```python
from build123d import *

# Parameters (mm, degrees)
SKETCH3_W           = 100
SKETCH3_H           = 63
BOSS_EXTRUDE1_DEPTH = 3
BOSS_EXTRUDE2_START = -3
SKETCH5_W           = 8
SKETCH5_H           = 6
BOSS_EXTRUDE2_DEPTH = 3
FILLET2_R           = 2
CUT_EXTRUDE1_DEPTH  = 3
CUT_EXTRUDE2_START  = -3
CUT_EXTRUDE2_DEPTH  = 3
CUT_EXTRUDE3_START  = -3
SKETCH8_W           = 39.05
SKETCH8_H           = 6
CUT_EXTRUDE3_DEPTH  = 3
SKETCH9_R           = 1.5
CUT_EXTRUDE4_DEPTH  = 10
FILL_PATTERN1_DEPTH = 3


# Read off the part's stored shape, not the designer's step: Cut-Extrude2, Fill Pattern1
with BuildPart() as part:
    # Sketch3 → Boss-Extrude1 (new body)
    with BuildSketch(Plane.XY):
        Rectangle(SKETCH3_W, SKETCH3_H)
    extrude(amount=BOSS_EXTRUDE1_DEPTH)

    # Sketch5 → Boss-Extrude2 (add)
    with BuildSketch(Plane(origin=(0, 0, 0), x_dir=(-1, 0, 0), z_dir=(0, 0, -1)).offset(BOSS_EXTRUDE2_START)):
        with Locations((-54, -28.5)):
            Rectangle(SKETCH5_W, SKETCH5_H)
        Polygon((-58, 29.5), (-50, 29.5), (-50, 31.5), (-48, 31.5), (-48, 35.5), (-58, 35.5), align=None)
        with Locations((54, -28.5)):
            Rectangle(SKETCH5_W, SKETCH5_H)
        Polygon((48, 35.5), (48, 31.5), (50, 31.5), (50, 29.5), (58, 29.5), (58, 35.5), align=None)
    extrude(amount=BOSS_EXTRUDE2_DEPTH)

    # Fillet2
    fillet2_edges = [part.edges().sort_by_distance(p)[0] for p in [
        (48, 35.5, 1.5),
        (58, 35.5, 1.5),
        (58, 29.5, 1.5),
        (50, 29.5, 1.5),
        (58, -31.5, 1.5),
        (58, -25.5, 1.5),
        (50, -25.5, 1.5),
        (-58, -31.5, 1.5),
        (-58, -25.5, 1.5),
        (-50, -25.5, 1.5),
        (-50, 29.5, 1.5),
        (-58, 29.5, 1.5),
        (-58, 35.5, 1.5),
        (-48, 35.5, 1.5),
        (-48, 31.5, 1.5),
        (48, 31.5, 1.5),
    ]]
    fillet(fillet2_edges, radius=FILLET2_R - 0.0001)  # a hair under: the kernel refuses the full size

    # Sketch6 → Cut-Extrude1 (cut)
    with BuildSketch(Plane.XY.offset(3)):
        with BuildLine():
            ThreePointArc((6.45, -3.15), (4.682233047, -3.882233047), (3.95, -5.65))
            Line((3.95, -5.65), (11.45, -5.65))
            Line((11.45, -5.65), (11.45, -3.15))
            Line((11.45, -3.15), (6.45, -3.15))
        make_face()
        with BuildLine():
            Line((11.45, -3.15), (11.45, -5.65))
            Line((11.45, -5.65), (18.95, -5.65))
            ThreePointArc((18.95, -5.65), (18.217766953, -3.882233047), (16.45, -3.15))
            Line((16.45, -3.15), (11.45, -3.15))
        make_face()
        with BuildLine():
            Line((18.95, -5.65), (11.45, -5.65))
            Line((11.45, -5.65), (11.45, -8.15))
            Line((11.45, -8.15), (16.45, -8.15))
            ThreePointArc((16.45, -8.15), (18.217766953, -7.417766953), (18.95, -5.65))
        make_face()
        with BuildLine():
            Line((11.45, -5.65), (3.95, -5.65))
            ThreePointArc((3.95, -5.65), (4.682233047, -7.417766953), (6.45, -8.15))
            Line((6.45, -8.15), (11.45, -8.15))
            Line((11.45, -8.15), (11.45, -5.65))
        make_face()
    extrude(amount=-CUT_EXTRUDE1_DEPTH, mode=Mode.SUBTRACT)

    # Cut-Extrude2 outline → Cut-Extrude2 (cut)
    with BuildSketch(Plane.XY.offset(3).offset(CUT_EXTRUDE2_START)):
        with BuildLine():
            Line((-11.2, 8.796347875), (-20.2, 8.796347875))
            ThreePointArc((-20.2, 8.796347875), (-22.2, 6.796347875), (-20.2, 4.796347875))
            Line((-20.2, 4.796347875), (1.9, 4.796347875))
            ThreePointArc((1.9, 4.796347875), (3.9, 6.796347875), (1.9, 8.796347875))
            Line((1.9, 8.796347875), (-11.19861108, 8.796347875))
            Line((-11.19861108, 8.796347875), (-11.2, 8.796347875))
        make_face()
    extrude(amount=CUT_EXTRUDE2_DEPTH, mode=Mode.SUBTRACT)

    # Sketch8 → Cut-Extrude3 (cut)
    with BuildSketch(Plane.XY.offset(3).offset(CUT_EXTRUDE3_START)):
        with BuildLine():
            Line((4.05, 14.6), (-35, 14.6))
            Line((-35, 14.6), (-35, 8.6))
            Line((-35, 8.6), (-21.064198479, 8.6))
            ThreePointArc((-21.064198479, 8.6), (-20.643111582, 8.746643269), (-20.2, 8.796347875))
            Line((-20.2, 8.796347875), (-11.2, 8.796347875))
            Line((-11.2, 8.796347875), (-11.19861108, 8.796347392))
            Line((-11.19861108, 8.796347392), (1.9, 8.796347875))
            ThreePointArc((1.9, 8.796347875), (2.343111582, 8.746643269), (2.764198479, 8.6))
            Line((2.764198479, 8.6), (4.05, 8.6))
            Line((4.05, 8.6), (4.05, 14.6))
        make_face()
        with BuildLine():
            ThreePointArc((-35, 20.6), (-39.242640687, 18.842640687), (-41, 14.6))
            Line((-41, 14.6), (-35, 14.6))
            Line((-35, 14.6), (-35, 20.6))
        make_face()
        with BuildLine():
            Line((-35, 14.6), (-41, 14.6))
            ThreePointArc((-41, 14.6), (-39.242640687, 10.357359313), (-35, 8.6))
            Line((-35, 8.6), (-35, 14.6))
        make_face()
        with Locations((-15.475, 17.6)):
            Rectangle(SKETCH8_W, SKETCH8_H)
        with BuildLine():
            Line((4.05, 20.6), (4.05, 14.6))
            Line((4.05, 14.6), (10.05, 14.6))
            ThreePointArc((10.05, 14.6), (8.292640687, 18.842640687), (4.05, 20.6))
        make_face()
        with BuildLine():
            Line((10.05, 14.6), (4.05, 14.6))
            Line((4.05, 14.6), (4.05, 8.6))
            ThreePointArc((4.05, 8.6), (8.292640687, 10.357359313), (10.05, 14.6))
        make_face()
    extrude(amount=CUT_EXTRUDE3_DEPTH, mode=Mode.SUBTRACT)

    # Sketch9 → Cut-Extrude4 (cut)
    with BuildSketch(Plane(origin=(0, 0, 0), x_dir=(-1, 0, 0), z_dir=(0, 0, -1))):
        with Locations((-54, 32.520438715)):
            Circle(SKETCH9_R)
        with Locations((54, 32.520438715)):
            Circle(SKETCH9_R)
        with Locations((-54, -28.5)):
            Circle(SKETCH9_R)
        with Locations((54, -28.5)):
            Circle(SKETCH9_R)
    extrude(amount=-CUT_EXTRUDE4_DEPTH, mode=Mode.SUBTRACT)

    # Fill Pattern1 outline → Fill Pattern1 (cut)
    with BuildSketch(Plane.XY):
        Polygon((34.648052979, 5.68067969), (32.648052979, 9.144781305), (28.648052979, 9.144781305), (26.648052979, 5.68067969), (28.648052979, 2.216578074), (32.648052979, 2.216578074), align=None)
        Polygon((27.719849748, 17.68067969), (25.719849748, 21.144781305), (21.719849748, 21.144781305), (19.719849748, 17.68067969), (21.719849748, 14.216578074), (25.719849748, 14.216578074), align=None)
        Polygon((35.576256209, 21.144781305), (33.576256209, 17.68067969), (35.576256209, 14.216578074), (39.576256209, 14.216578074), (41.576256209, 17.68067969), (39.576256209, 21.144781305), align=None)
        Polygon((34.648052979, 21.68067969), (32.648052979, 25.144781305), (28.648052979, 25.144781305), (26.648052979, 21.68067969), (28.648052979, 18.216578074), (32.648052979, 18.216578074), align=None)
        Polygon((41.576256209, 9.68067969), (39.576256209, 13.144781305), (35.576256209, 13.144781305), (33.576256209, 9.68067969), (35.576256209, 6.216578074), (39.576256209, 6.216578074), align=None)
        Polygon((21.719849748, 13.144781305), (19.719849748, 9.68067969), (21.719849748, 6.216578074), (25.719849748, 6.216578074), (27.719849748, 9.68067969), (25.719849748, 13.144781305), align=None)
        Polygon((34.648052979, 13.68067969), (32.648052979, 17.144781305), (28.648052979, 17.144781305), (26.648052979, 13.68067969), (28.648052979, 10.216578074), (32.648052979, 10.216578074), align=None)
    extrude(amount=FILL_PATTERN1_DEPTH, mode=Mode.SUBTRACT)


solid = part.part
```
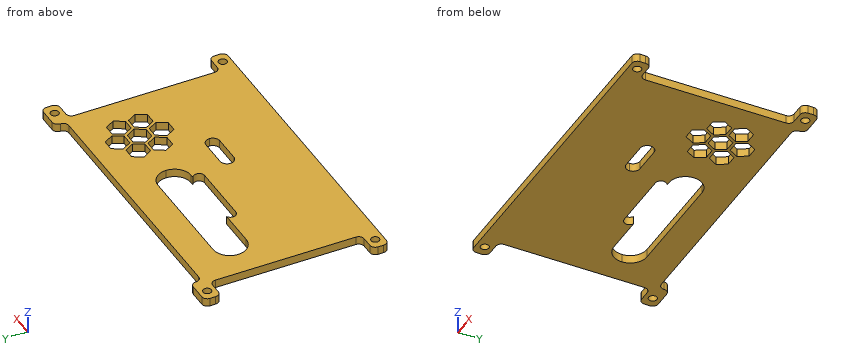
The listing builds one solid part. Answer for the finished solid, in the listing's coordinates (mm). Round coordinates to 2 decimals unless told otherwise and drop trailing zeros. Loops run counter-clockwise (first coordinate to the right, second up) from the corner with the lowest first, then second, coordinate; pieces in that order, holes last. Notation, with made-up numbers: (64.25, 53.5) -> (106.25, 53.5) arc R27 cw to (106.25, 73.5) -> close; hole circle Ø1 at (89.25, -36). An arc over 180 degrees is marked (long way). Use one line per item in the form item = value.
1. Find the intervals of material crossed by probe 1 along Y at (x, z) = (-54, 1.6); probe 2 along Y at (x, z) = (-34, 0.7); probe 3 along Y at (x, z) = (13, 2.35), in increasing order. Write a range as [from, to].
Answer key:
probe_1 = [-31.5, -30], [-27, -25.5], [29.5, 31.02], [34.02, 35.5]
probe_2 = [-31.5, 8.6], [20.6, 31.5]
probe_3 = [-31.5, -8.15], [-3.15, 31.5]
2. The part is cut by section C-C on x = 38.5. Determine the outline of the cut face in (y, z).
Answer key:
outline = (-31.5, 0) -> (6.22, 0) -> (6.22, 3) -> (-31.5, 3) -> close; (13.14, 0) -> (14.22, 0) -> (14.22, 3) -> (13.14, 3) -> close; (21.14, 0) -> (31.5, 0) -> (31.5, 3) -> (21.14, 3) -> close
3. The part is cut by section B-B on x = -19. Determine the outline of the cut face in (y, z), and give its area (3 significant figures).
Answer key:
outline = (-31.5, 0) -> (4.8, 0) -> (4.8, 3) -> (-31.5, 3) -> close; (20.6, 0) -> (31.5, 0) -> (31.5, 3) -> (20.6, 3) -> close
area = 142 mm²
4. The part is cut by section D-D on y = 23.5. Determine the outline of the cut face in (x, z), and give its area (3 significant figures).
Answer key:
outline = (-50, 0) -> (27.7, 0) -> (27.7, 3) -> (-50, 3) -> close; (33.6, 0) -> (50, 0) -> (50, 3) -> (33.6, 3) -> close
area = 282 mm²
5. Flat-ended cylindrical pins translate along their axes: pin 1 Ø1.5 at (x, z) = (38, 2) entering from +Y; pin 2 Ø1.8 at (x, y) = (-54, 32.52) entering from +Z. Find the tip coordinate at first contact, or state that the pin passes through.
Answer key:
pin_1 = 31.5
pin_2 = through
6. The part is cut by section A-A on x = 54. Determine the outline of the cut face in (y, z), and give its area (3 significant figures).
Answer key:
outline = (-31.5, 0) -> (-30, 0) -> (-30, 3) -> (-31.5, 3) -> close; (-27, 0) -> (-25.5, 0) -> (-25.5, 3) -> (-27, 3) -> close; (29.5, 0) -> (31.02, 0) -> (31.02, 3) -> (29.5, 3) -> close; (34.02, 0) -> (35.5, 0) -> (35.5, 3) -> (34.02, 3) -> close
area = 18.0 mm²
